Source: CAD feature listing. Evaluate the final solid. Frame: model axes, mm. A direction names the side the tool comes from. Give positions to 0.01 mm unless a question says otherwise; leave off trailing zeros. Write each loop counter-clockwise with the first axis right and the second up, starting at its lowest first coordinate (ties: lowest second). Pieces come first, ordered by that corner, then holes.
```python
from build123d import *

# Parameters (mm, degrees)
F1_DEPTH      = 50
F1_DEPTH_BACK = 70
F2_SIZE       = 25
F4_DEPTH      = 25
F6_DEPTH      = 25
F7_W          = 9.5013230816
F7_H          = 6.2035092162
F8_DEPTH      = 150
F8_DEPTH_BACK = 150
F9_W          = 6.2035092162
F9_H          = 120
F10_DEPTH     = 0.5


with BuildPart() as f1:
    # F0 (on Top) → F1 (new body, two sides)
    with BuildSketch(Plane.XY) as f1_sk:
        with BuildLine():
            Line((-133.4287243432, 183.7437768202), (-138.188844385, 180.0912082461))
            Line((-138.188844385, 180.0912082461), (-4.7601200417, 6.2035092162))
            ThreePointArc((-4.7601200417, 6.2035092162), (0, 3.8560777902), (4.7601200417, 6.2035092162))
            Line((4.7601200417, 6.2035092162), (138.188844385, 180.0912082461))
            Line((138.188844385, 180.0912082461), (133.4287243432, 183.7437768202))
            Line((133.4287243432, 183.7437768202), (2.3800600209, 12.9578323983))
            ThreePointArc((2.3800600209, 12.9578323983), (0, 11.7841166853), (-2.3800600209, 12.9578323983))
            Line((-2.3800600209, 12.9578323983), (-133.4287243432, 183.7437768202))
        make_face()
    extrude(amount=F1_DEPTH)
    extrude(f1_sk.sketch, amount=-F1_DEPTH_BACK)

    # F2
    f2_edges = [f1.edges().sort_by_distance(p)[0] for p in [
        (-135.808784, 181.917493, 50),
        (135.808784, 181.917493, 50),
    ]]
    chamfer(f2_edges, length=F2_SIZE)

    # F3 (on face) → F4 (cut)
    with BuildSketch(Plane(origin=(0, 0, 0), x_dir=(0.608761429, -0.7933533403, 0), z_dir=(-0.7933533403, -0.608761429, 0))):
        Polygon((-66.5563264195, 0), (-227, 0), (-227, -70), (-7.819352237, -70), align=None)
    extrude(amount=-F4_DEPTH, mode=Mode.SUBTRACT)

    # F5 (on face) → F6 (cut)
    with BuildSketch(Plane(origin=(0, 0, 0), x_dir=(0.608761429, 0.7933533403, 0), z_dir=(0.7933533403, -0.608761429, 0))):
        Polygon((66.5563264195, 0), (7.819352237, -70), (227, -70), (227, 0), align=None)
    extrude(amount=-F6_DEPTH, mode=Mode.SUBTRACT)

    # F7 (on Top) → F8 (cut, two sides)
    with BuildSketch(Plane.XY) as f8_sk:
        with Locations((-0.0094585009, 3.1017546081)):
            Rectangle(F7_W, F7_H)
    extrude(amount=F8_DEPTH, mode=Mode.SUBTRACT)
    extrude(f8_sk.sketch, amount=-F8_DEPTH_BACK, mode=Mode.SUBTRACT)

    # F9 (on Right) → F10 (join, symmetric)
    with BuildSketch(Plane.YZ):
        with Locations((3.1017546081, -10)):
            Rectangle(F9_W, F9_H)
    extrude(amount=F10_DEPTH, both=True)


solid = f1.part
```
1. Line query: probe 1 along X at (y, z) = (39, -8); probe 2 along X at (y, z) = (86, 33); probe 3 along Y at (x, z) = (-117.5, 12). Output: solid intervals per line, ascending.
2. Section query B-B (y = 31.5). Return loops of the section in (x, z).
3. Section query C-C (y = 146). Return loops of the section in (x, z), plus the area to 3 significant figures.
4. Access query for faces 1 (the flat face through (0.5, 3, -9)), 2 (the flat face through (-0.5, 3, -9)), 3 (the flat face through (54.26, 80.57, 18.77)), 4 (the flat face through (-128.06, 171.89, 37.67)). Directions: +Z, -Z, +X, -X, +Y, -Y. A direction counts if a zero-diameter tool reaches every point of the face in a straight line with its end or side. Return the directions, or none.
5. Pin query (flat end, axial travel): P1, Ø5, axis at y = 91.5, z = 23, coming from the +X side; P2, Ø1.5, axis at y = 74.5, z = 9.5, coming from the +X side; P3, Ø6, axis at y = 37.5, z = -6, coming from the +X side. Return the tip coordinate at first contact, or that it passes through.
The answers:
1. probe 1: x = -29.93 to -22.36, 22.36 to 29.93
1. probe 2: x = -65.99 to -58.43, 58.43 to 65.99
1. probe 3: y = 153.13 to 162.99
2. outline: (-24.17, -32) - (-16.61, -37.49) - (-16.61, 50) - (-24.17, 50) - close; (16.61, -37.49) - (24.17, -32) - (24.17, 50) - (16.61, 50) - close
3. outline: (-112.03, 0) - (-104.47, 0) - (-104.47, 50) - (-112.03, 50) - close; (104.47, 0) - (112.03, 0) - (112.03, 50) - (104.47, 50) - close
3. area: 756 mm2
4. face 1: +Z, -Z, +X, -Y
4. face 2: +Z, -Z, -X, -Y
4. face 3: +Z, -Z, +Y
4. face 4: +Z, -X, +Y
5. P1: stops at x = 72.13
5. P2: stops at x = 57.74
5. P3: stops at x = 31.08
